```python
from build123d import *

# Parameters (mm, degrees)
SKETCH1_W           = 38.1
SKETCH1_H           = 73.66
SKETCH1_R           = 4.5212
SKETCH1_W_2         = 27.94
SKETCH1_H_2         = 5.08
BOSS_EXTRUDE1_DEPTH = 3.175
FILLET1_R           = 5.08
FILLET2_R           = 1.27


with BuildPart() as part:
    # Sketch1 → Boss-Extrude1 (new body)
    with BuildSketch(Plane(origin=(0, 0, 0), x_dir=(1, 0, 0), z_dir=(0, 1, 0))):
        with Locations((0, -24.13)):
            Rectangle(SKETCH1_W, SKETCH1_H)
        with Locations(Location((0, 0, 0), (0, 0, 270))):  # turned: the seam where the file's is
            Circle(SKETCH1_R, mode=Mode.SUBTRACT)
        with Locations((0, -53.34)):
            Rectangle(SKETCH1_W_2, SKETCH1_H_2, mode=Mode.SUBTRACT)
    extrude(amount=BOSS_EXTRUDE1_DEPTH)

    # Fillet1
    fillet1_edges = [part.edges().sort_by_distance(p)[0] for p in [
        (-19.05, 1.5875, -12.7),
        (19.05, 1.5875, -12.7),
        (19.05, 1.5875, 60.96),
        (-19.05, 1.5875, 60.96),
    ]]
    fillet(fillet1_edges, radius=FILLET1_R)

    # Fillet2
    fillet2_edges = [part.edges().sort_by_distance(p)[0] for p in [
        (-13.97, 1.5875, 50.8),
        (-13.97, 1.5875, 55.88),
        (13.97, 1.5875, 55.88),
        (13.97, 1.5875, 50.8),
    ]]
    fillet(fillet2_edges, radius=FILLET2_R)


solid = part.part
```
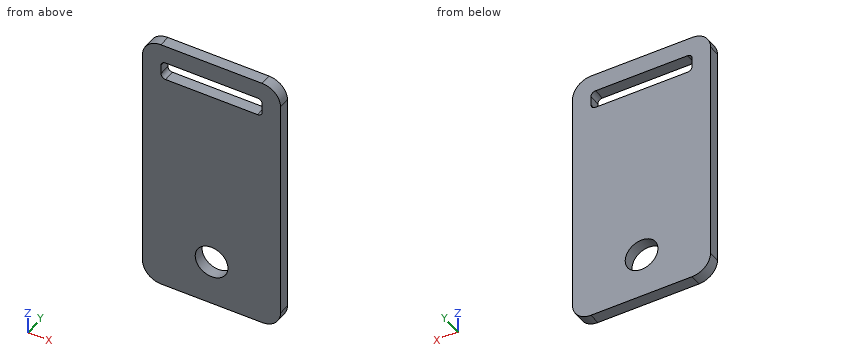
For this review, take the finished solid that the model builds, in its own axes (mm). Give positions to 0.01 mm unless a question says otherwise; leave off trailing zeros. Write each loop counter-clockwise with the first axis right and the second up, starting at its lowest first coordinate (ties: lowest second). Pieces come first, ordered by that corner, then holes. Notation, with made-up numbers: M 73,-7 L 89,-7 A25 cw 89,21 Z; hole C -21,78.25 d7. An arc over 180 degrees is marked long. Answer as CSV lines item,"result".
1. For pin 1 (8 mm diameter, centred on x = 0, z = 0, fed in from -Y), flat-tipped, find the tip position at first contact; note if it passes through.
Findings:
pin 1,"passes through"
2. Wall thickness on line 1 (Z direction, x = 10, y = 1.95); line 2 (X direction, y = 1.65, z = 0); line 3 (Z direction, x = -0.5, y = 1.6): over which ranges is each line inside the solid? List them lowest first.
Findings:
line 1,"z = -12.7 to 50.8, 55.88 to 60.96"
line 2,"x = -19.05 to -4.52, 4.52 to 19.05"
line 3,"z = -12.7 to -4.49, 4.49 to 50.8, 55.88 to 60.96"
3. Consider section B-B, the plane y = 0.65. Write out the cut boundary in (x, z), then the cut area to 3 significant figures.
Findings:
outline,"M -19.05,-7.62 A5.08 ccw -13.97,-12.7 L 13.97,-12.7 A5.08 ccw 19.05,-7.62 L 19.05,55.88 A5.08 ccw 13.97,60.96 L -13.97,60.96 A5.08 ccw -19.05,55.88 Z; hole M -13.97,52.07 A1.27 ccw -12.7,50.8 L 12.7,50.8 A1.27 ccw 13.97,52.07 L 13.97,54.61 A1.27 ccw 12.7,55.88 L -12.7,55.88 A1.27 ccw -13.97,54.61 Z; hole C 0,0 d9.04"
area,"2,580 mm2"
4. Consider section D-D, the plane x = -10.5. Write out the cut boundary in (y, z) (3 decimals), then the cut area to 3 significant figures.
Findings:
outline,"M 0,-12.7 L 3.175,-12.7 L 3.175,50.8 L 0,50.8 Z; M 0,55.88 L 3.175,55.88 L 3.175,60.96 L 0,60.96 Z"
area,"218 mm2"
5. Consider section C-C, the plane z = 0. Write out the cut boundary in (x, y) (3 decimals).
Findings:
outline,"M -19.05,0 L -4.521,0 L -4.521,3.175 L -19.05,3.175 Z; M 4.521,0 L 19.05,0 L 19.05,3.175 L 4.521,3.175 Z"
6. Consider section A-A, the plane x = 0. Write out the cut boundary in (y, z) (3 decimals).
Findings:
outline,"M 0,-12.7 L 3.175,-12.7 L 3.175,-4.521 L 0,-4.521 Z; M 0,4.521 L 3.175,4.521 L 3.175,50.8 L 0,50.8 Z; M 0,55.88 L 3.175,55.88 L 3.175,60.96 L 0,60.96 Z"
